Autodesk Inventor part; units mm, degrees
ref_plane "YZ Plane" through (0, 0, 0) normal (1, 0, 0) x (0, 1, 0)
ref_plane "XZ Plane" through (0, 0, 0) normal (0, 1, 0) x (-1, 0, 0)
ref_plane "XY Plane" through (0, 0, 0) normal (0, 0, 1) x (1, 0, 0)
sketch "Sketch1" plane through (0, 0, 0) normal (0, 0, 1) x (1, 0, 0)
  line L0 (-1.8974, -23.3494) -> (-1.8974, -74.3026)
  line L1 (-1.8974, -74.3026) -> (0, -74.3026)
  line L2 (0, -74.3026) -> (0, 0)
  line L3 (0, 0) -> (99.7026, 0)
  line L4 (99.7026, 0) -> (99.7026, 1.8974)
  line L5 (99.7026, 1.8974) -> (-1.8974, 1.8974)
  line L6 (-1.8974, 1.8974) -> (-1.8974, -23.3494)
  dimension "d0" = 101.6
  dimension "d1" = 76.2
  dimension "d2" = 1.8974
  dimension "d3" = 1.8974
extrude "Extrusion1" add sketch "Sketch1" against normal blind 2159
sketch "Sketch2" plane through (0, -74.3026, 0) normal (1, 0, 0) x (0, 0, -1)
  line L0 (2159, 74.3026) -> (2159, 0)
  line L1 (2159, 74.3026) -> (2139.0907, 0)
  line L2 (0, 0) -> (2159, 0)
  line L3 (2139.0907, 0) -> (2159, 0)
  line L4 (2159, 0) -> (2159, 74.3026)
  point P0 (0, 74.3026)
  dimension "d9" = 15
extrude "Extrusion3" cut sketch "Sketch2" against normal up to next
properties part number "Angle--Back"
Could you check a few things on this model? Use its own coordinates, in mm. Give positions to 0.01 mm unless a question says otherwise; leave off trailing zeros. Order: outer loops, then holes, each group sorted by start corner. A loop starts at its lowest first (then second) coordinate and runs counter-clockwise, first axis right, second up. Notation, with made-up numbers: (52.25, 35) -> (62.25, 35) arc R27 cw to (62.25, 62) -> close; hole circle Ø5 at (-11, 73.5). An arc over 180 degrees is marked (long way). Return JSON: item names as keys, results as strings.
1. For pin 1 Ø2 at (x, z) = (52.5, -436.5) entering from -Y, with a flat end and sliding along its axis, tell me the tip position at first contact or that it passes through.
Answer list:
{"pin 1": "stops at y = 0"}
2. I need wall thicknesses on line 1 (Y direction, x = 72.5, z = -1779.5); line 2 (X direction, y = -69, z = -775). Which ranges of each line are inside material? Lowest first, please. Write a range as from..to.
Answer list:
{"line 1": "y = 0..1.9", "line 2": "x = -1.9..0"}
3. Imagine slicing it at A-A on z = -160. List the corners of the cut face in (x, y) for me, then the cut area to 3 significant figures.
Answer list:
{"outline": "(-1.9, -74.3) -> (0, -74.3) -> (0, 0) -> (99.7, 0) -> (99.7, 1.9) -> (-1.9, 1.9) -> close", "area": "334 mm2"}
4. Imagine slicing it at B-B on x = 36.5. List the corners of the cut face in (y, z) for me.
Answer list:
{"outline": "(0, -2159) -> (1.9, -2159) -> (1.9, 0) -> (0, 0) -> close"}
5. Thinking about a two-plate mould opening in X: for faces 1 (the flat face through (49, 0, -1064)), 2 (the flat face through (0, -38, -1064)), 3 (the flat face through (-1.897, -36, -1064)), which applies, pulls with the +X half, pulls with the -X half, needs draft (parallel to the pull), parting line crosses it, or undercut?
Answer list:
{"face 1": "needs draft", "face 2": "pulls with the +X half", "face 3": "pulls with the -X half"}
6. Imagine slicing it at C-C on y = -47.5. List the corners of the cut face in (x, z) for me.
Answer list:
{"outline": "(-1.9, -2146.27) -> (0, -2146.27) -> (0, 0) -> (-1.9, 0) -> close"}
